from build123d import *

# Parameters (mm, degrees)
BODYTOP_R                       = 19
BODY_TOP_DEPTH                  = 1
SKIZZE_LAMELLEN_W               = 1.2
SKIZZE_LAMELLEN_H               = 85
LAMMELLEN_DEPTH                 = 2.5
SKIZZE1_W                       = 1.9
SKIZZE1_H                       = 85
FUEHRUNG_DEPTH                  = 1.5
VERRUNDUNG6_R                   = 1
SPARUNG_W                       = 1.2
SPARUNG_H                       = 30
AUSSPARUNG_DEPTH                = 2.5
ANBAUPLATTE_DEPTH               = 1
ANBAUSTUTZEN_DEPTH              = 15.5
SKIZZEDRUCKERZAHNRAD_R          = 3.75
SKIZZEDRUCKERZAHNRAD_R_2        = 3
DRUCKER_ZAHNRAD_DEPTH           = 2
SKIZZEHALTERLOCH_R              = 2.1
HALTERLOCH_DEPTH                = 18.5
VERRUNDUNG24_R                  = 8
SKIZZEBOHRLOCH_R                = 0.9
BOHRLOCH_DEPTH                  = 10
SKIZZE6_W                       = 7.001894066
SKIZZE6_H                       = 6.469061082
SKIZZE6_W_2                     = 3.181141547
SCHNITT_LINEAR_AUSTRAGEN4_DEPTH = 15.5
VERRUNDUNG34_R                  = 1
SCHNITT_LINEAR_START            = -18.5000001
SCHNITT_LINEAR_AUSTRAGEN5_DEPTH = 19.5000002
LINEARES_MUSTER2_COUNT          = 11
LINEARES_MUSTER2_PITCH          = 8
SCHNITT_LINEAR_START_2          = -3.0000001
SCHNITT_LINEAR_AUSTRAGEN6_DEPTH = 19.5000002
KREISMUSTER1_COUNT              = 9
VERRUNDUNG35_R                  = 2
VERRUNDUNG36_R                  = 4
VERRUNDUNG37_R                  = 4
VERRUNDUNG38_R                  = 0.75


with BuildPart() as part:
    # BodyTop → body-top (new body, symmetric)
    with BuildSketch(Plane.XY):
        Circle(BODYTOP_R)
        with BuildLine():
            ThreePointArc((19, 0), (13.435028843, -13.435028843), (0, -19))
            Line((0, -19), (27, -19))
            Line((27, -19), (27, 66))
            Line((27, 66), (7, 66))
            Line((7, 66), (7, 19))
            Line((7, 19), (0, 19))
            ThreePointArc((0, 19), (13.435028843, 13.435028843), (19, 0))
        make_face()
    extrude(amount=BODY_TOP_DEPTH, both=True)

    # skizze_lamellen → Lammellen (add)
    with BuildSketch(Plane.XY.offset(1)):
        with Locations((24, 23.5)):
            Rectangle(SKIZZE_LAMELLEN_W, SKIZZE_LAMELLEN_H)
        with Locations((10, 23.5)):
            Rectangle(SKIZZE_LAMELLEN_W, SKIZZE_LAMELLEN_H)
    extrude(amount=LAMMELLEN_DEPTH)

    # Skizze1 → fuehrung (add)
    with BuildSketch(Plane.XY.offset(1)):
        with Locations((15.15, 23.5)):
            Rectangle(SKIZZE1_W, SKIZZE1_H)
    extrude(amount=FUEHRUNG_DEPTH)

    # Verrundung6
    verrundung6_edges = [part.edges().sort_by_distance(p)[0] for p in [
        (27, -19, 0),
    ]]
    fillet(verrundung6_edges, radius=VERRUNDUNG6_R)

    # sparung → Aussparung (cut)
    with BuildSketch(Plane.XY.offset(3.5)):
        with Locations((10, 0.5)):
            Rectangle(SPARUNG_W, SPARUNG_H)
    extrude(amount=-AUSSPARUNG_DEPTH, mode=Mode.SUBTRACT)

    # SkizzeAnbau → Anbauplatte (add, symmetric)
    with BuildSketch(Plane.XY):
        with BuildLine():
            Line((7, 74), (7, 66))
            Line((7, 66), (27, 66))
            Line((27, 66), (27, 74))
            ThreePointArc((27, 74), (17, 84), (7, 74))
        make_face()
    extrude(amount=ANBAUPLATTE_DEPTH, both=True)

    # SkizzeStutzen → anbaustutzen (add)
    with BuildSketch(Plane.XY.offset(1)):
        with BuildLine():
            Line((7, 66), (27, 66))
            Line((27, 66), (27, 74))
            ThreePointArc((27, 74), (17, 84), (7, 74))
            Line((7, 74), (7, 66))
        make_face()
    extrude(amount=ANBAUSTUTZEN_DEPTH)

    # Skizzedruckerzahnrad → drucker zahnrad (add)
    with BuildSketch(Plane.XY.offset(1)):
        Circle(SKIZZEDRUCKERZAHNRAD_R)
        Circle(SKIZZEDRUCKERZAHNRAD_R_2, mode=Mode.SUBTRACT)
    extrude(amount=DRUCKER_ZAHNRAD_DEPTH)

    # SkizzeHalterloch → halterloch (cut)
    with BuildSketch(Plane.XY.offset(16.5)):
        with Locations((17, 77)):
            Circle(SKIZZEHALTERLOCH_R)
    extrude(amount=-HALTERLOCH_DEPTH, mode=Mode.SUBTRACT)

    # Verrundung24
    verrundung24_edges = [part.edges().sort_by_distance(p)[0] for p in [
        (7, 19, 0),
    ]]
    fillet(verrundung24_edges, radius=VERRUNDUNG24_R)

    # Skizzebohrloch → bohrloch (cut)
    with BuildSketch(Plane.XY.offset(1)):
        with Locations((7.4, -17.5)):
            Circle(SKIZZEBOHRLOCH_R)
        with Locations((6.1, 19.2)):
            Circle(SKIZZEBOHRLOCH_R)
    extrude(amount=-BOHRLOCH_DEPTH, mode=Mode.SUBTRACT)

    # Skizze6 → Schnitt-Linear austragen4 (cut)
    with BuildSketch(Plane.XY.offset(16.5)):
        with Locations((19.600947033, 69.234530541)):
            Rectangle(SKIZZE6_W, SKIZZE6_H)
        with Locations((12.609429227, 69.234530541)):
            Rectangle(SKIZZE6_W_2, SKIZZE6_H)
    extrude(amount=-SCHNITT_LINEAR_AUSTRAGEN4_DEPTH, mode=Mode.SUBTRACT)

    # Verrundung34
    verrundung34_edges = [part.edges().sort_by_distance(p)[0] for p in [
        (15.15, -19, 2.5),
    ]]
    fillet(verrundung34_edges, radius=VERRUNDUNG34_R)

    # Skizze7 → Schnitt-Linear austragen5 (cut)
    with BuildSketch(Plane(origin=(0, 0, -1), x_dir=(-1, 0, 0), z_dir=(0, 0, -1)).offset(SCHNITT_LINEAR_START)):
        Polygon((-22.413127148, -12.56760803), (-21.225184268, -14.625185455), (-18.849298507, -14.625185455), (-17.661355626, -12.56760803), (-18.849298507, -10.510030604), (-21.225184268, -10.510030604), align=None)
    schnitt_linear_austragen5 = extrude(amount=SCHNITT_LINEAR_AUSTRAGEN5_DEPTH, mode=Mode.SUBTRACT)

    # Lineares Muster2: Schnitt-Linear austragen5 ×11
    with Locations(*[(0, i * LINEARES_MUSTER2_PITCH, 0) for i in range(1, LINEARES_MUSTER2_COUNT)]):
        add(schnitt_linear_austragen5, mode=Mode.SUBTRACT)

    # Skizze8 → Schnitt-Linear austragen6 (cut)
    with BuildSketch(Plane.XY.offset(1).offset(SCHNITT_LINEAR_START_2)):
        Polygon((0, -8.844754272), (-2.078547165, -10.044804037), (-2.078547165, -12.444903567), (0, -13.644953333), (2.078547165, -12.444903567), (2.078547165, -10.044804037), align=None)
    schnitt_linear_austragen6 = extrude(amount=SCHNITT_LINEAR_AUSTRAGEN6_DEPTH, mode=Mode.SUBTRACT)

    # Kreismuster1: Schnitt-Linear austragen6 ×9 about axis
    kreismuster1_axis = Axis((0, 0, 0), (0, 0, 1))
    for i in range(1, KREISMUSTER1_COUNT):
        add(schnitt_linear_austragen6.rotate(kreismuster1_axis, i * 360 / KREISMUSTER1_COUNT), mode=Mode.SUBTRACT)

    # Verrundung35
    verrundung35_edges = [part.edges().sort_by_distance(p)[0] for p in [
        (23.101894066, 72.469061082, 8.75),
    ]]
    fillet(verrundung35_edges, radius=VERRUNDUNG35_R)

    # Verrundung36
    verrundung36_edges = [part.edges().sort_by_distance(p)[0] for p in [
        (10, 66, 3.5),
    ]]
    fillet(verrundung36_edges, radius=VERRUNDUNG36_R)

    # Verrundung37
    verrundung37_edges = [part.edges().sort_by_distance(p)[0] for p in [
        (24, 66, 3.5),
    ]]
    fillet(verrundung37_edges, radius=VERRUNDUNG37_R)

    # Verrundung38
    verrundung38_edges = [part.edges().sort_by_distance(p)[0] for p in [
        (10, 15.5, 3.5),
        (10, -19, 3.5),
        (24, -19, 3.5),
    ]]
    fillet(verrundung38_edges, radius=VERRUNDUNG38_R)


solid = part.part
Design review of the part built by this model. Coordinates are the model's own, in mm. A direction names the side the tool comes from. Coordinates: 2 decimals unless noted, no trailing zeros. Order: outer loops, then holes, each group sorted by start corner. A loop starts at its lowest first (then second) coordinate and runs counter-clockwise, first axis right, second up. Notation, with made-up numbers: (-24.75, -13) - (-19.75, -13) arc R25 cw to (-19.75, 5) - close; hole circle Ø1 at (50.5, 85.25). An arc over 180 degrees is marked (long way). Put each result on its own line as item: value.
1) The part is to be moulded in two halves that separate along X. For faces 5 (the face through (26, 24, 1)), 6 (the face through (21.83, 42.42, 0.01)), say which applies: released by +X, released by -X, zero draft, split by the parting line, or undercut.
Response values:
face 5: zero draft
face 6: undercut
2) Tool access review of faces 1 (the face through (1.05, -9.45, -0.01)), 2 (the face through (24.008, 64.859, 4.703)), 3 (the face through (0, 0, 1)), 4 (the face through (14.2, 43, 2)): name each direction out of +Z, -Z, +X, -X, +Y, -Y from which nothing blocks a thin tool from reaching the whole face with its end or side.
Response values:
face 1: +Z, -Z
face 2: +Z, +X, -X, -Y
face 3: +Z
face 4: +Z, -Y
3) Wall thickness on L1, parallel to X at y = 69, z = 10.75; L2, parallel to Y at x = 17, z = 4.25; L3, parallel to Z at x = 25, y = -3: over which ranges is each line inside the solid? List them lowest first. Write a range as from..to.
Response values:
L1: x = 7..11.02, 14.2..16.1, 23.1..27
L2: y = 72.47..74.9, 79.1..84
L3: z = -1..1
4) Take a section at A-A, the plane z = 15. Give the boundary of the cut face in (x, y), and give its area (3 significant figures).
Response values:
outline: (7, 66) - (11.02, 66) - (11.02, 72.47) - (14.2, 72.47) - (14.2, 66) - (16.1, 66) - (16.1, 72.47) - (21.1, 72.47) arc R2 cw to (23.1, 70.47) - (23.1, 66) - (27, 66) - (27, 74) arc R10 ccw to (7, 74) - close; hole circle Ø4.2 at (17, 77)
area: 238 mm²
5) Insertion check: P1, Ø12, axis at x = -10, y = -6, coming from the +Z side; P2, Ø12, axis at x = 0, y = 47, coming from the +Z side; P3, Ø3, axis at x = 11, z = 14, coming from the -Y side; P4, Ø3, axis at y = -17, z = 2, coming from the -X side. Each pin has a flat end and moves straight along its axis. Give the tip position at first contact, or say it passes through.
Response values:
P1: stops at z = 1
P2: passes through
P3: stops at y = 66
P4: stops at x = -10.43
6) Take a section at C-C, the plane z = 0. Count the separate pieces of the cut face and the enclosed holes in it, and give its area (3 significant figures).
Response values:
separate pieces: 1
enclosed holes: 23
area: 2,550 mm²
7) Take a section at B-B, the plane y = 77. Give the boundary of the cut face in (x, z).
Response values:
outline: (7.46, -1) - (14.9, -1) - (14.9, 16.5) - (7.46, 16.5) - close; (19.1, -1) - (26.54, -1) - (26.54, 16.5) - (19.1, 16.5) - close
